Design review of the part built by this model. Coordinates are the model's own, in mm. Face numbers are marked on the shaded views. A direction names the side the tool comes from. Give positions to 0.01 mm unless a question says otherwise; leave off trailing zeros. Loops run counter-clockwise (first coordinate to the right, second up) from the corner with the lowest first, then second, coordinate; pieces in that order, holes last. Notation, with made-up numbers: (9.25, -21.5) - (43.25, -21.5) arc R13 ccw to (43.25, -4.5) - close; hole circle Ø11 at (-32.75, -24.75). An arc over 180 degrees is marked (long way). Write each question's results on one line, items separated by ' | '.
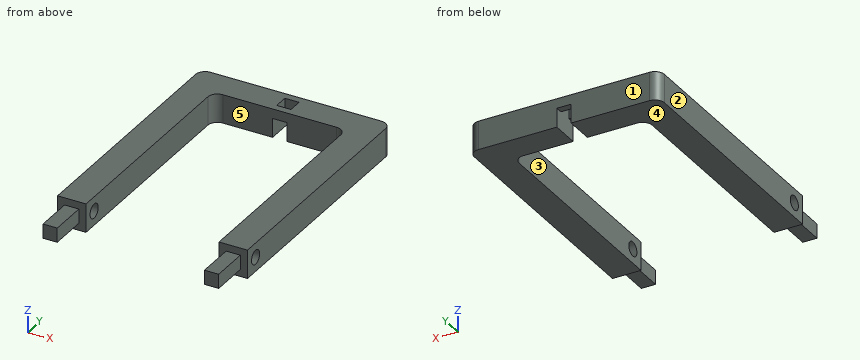
from build123d import *

# Parameters (mm, degrees)
BOSS_EXTRUDE1_DEPTH     = 30
SKETCH2_W               = 15
SKETCH2_H               = 15
BOSS_EXTRUDE2_DEPTH     = 40
FILLET1_R               = 10
FILLET2_R               = 10
SKETCH3_R               = 7.5
CUT_EXTRUDE1_DEPTH      = 171
CUT_EXTRUDE1_DEPTH_BACK = 31
SKETCH4_W               = 15
SKETCH4_H               = 30
CUT_EXTRUDE2_DEPTH      = 20
SKETCH5_W               = 15
SKETCH5_H               = 15
CUT_EXTRUDE3_DEPTH      = 10


with BuildPart() as part:
    # Sketch1 → Boss-Extrude1 (new body)
    with BuildSketch(Plane.XY):
        Polygon((-77.931034483, -87.881800857), (-107.931034483, -87.881800857), (-107.931034483, 177.118199143), (92.068965517, 177.118199143), (92.068965517, -87.881800857), (62.068965517, -87.881800857), (62.068965517, 147.118199143), (-77.931034483, 147.118199143), align=None)
    extrude(amount=BOSS_EXTRUDE1_DEPTH)

    # Sketch2 → Boss-Extrude2 (add)
    with BuildSketch(Plane.XZ.offset(87.881800857)):
        with Locations((77.068965517, 15)):
            Rectangle(SKETCH2_W, SKETCH2_H)
        with Locations((-92.931034483, 15)):
            Rectangle(SKETCH2_W, SKETCH2_H)
    extrude(amount=BOSS_EXTRUDE2_DEPTH)

    # Fillet1
    fillet1_edges = [part.edges().sort_by_distance(p)[0] for p in [
        (62.068965517, 147.118199143, 15),
        (-77.931034483, 147.118199143, 15),
    ]]
    fillet(fillet1_edges, radius=FILLET1_R)

    # Fillet2
    fillet2_edges = [part.edges().sort_by_distance(p)[0] for p in [
        (-107.931034483, 177.118199143, 15),
        (92.068965517, 177.118199143, 15),
    ]]
    fillet(fillet2_edges, radius=FILLET2_R)

    # Sketch3 → Cut-Extrude1 (cut, two sides)
    with BuildSketch(Plane(origin=(-77.931034483, 0, 0), x_dir=(0, 0, -1), z_dir=(1, 0, 0))) as cut_extrude1_sk:
        with Locations((-15, -72.881800857)):
            Circle(SKETCH3_R)
    extrude(amount=CUT_EXTRUDE1_DEPTH, mode=Mode.SUBTRACT)
    extrude(cut_extrude1_sk.sketch, amount=-CUT_EXTRUDE1_DEPTH_BACK, mode=Mode.SUBTRACT)

    # Sketch4 → Cut-Extrude2 (cut)
    with BuildSketch(Plane(origin=(0, 0, 0), x_dir=(-1, 0, 0), z_dir=(0, 0, -1))):
        with Locations((7.930867489, 162.118199143)):
            Rectangle(SKETCH4_W, SKETCH4_H)
    extrude(amount=-CUT_EXTRUDE2_DEPTH, mode=Mode.SUBTRACT)

    # Sketch5 → Cut-Extrude3 (cut)
    with BuildSketch(Plane.XY.offset(30)):
        with Locations((-7.930867489, 162.118199143)):
            Rectangle(SKETCH5_W, SKETCH5_H)
    extrude(amount=-CUT_EXTRUDE3_DEPTH, mode=Mode.SUBTRACT)


solid = part.part
(1) Take a section at A-A on y = -15.5. Give the boundary of the cut face in (x, z).
Answers below:
outline: (-107.93, 0) - (-77.93, 0) - (-77.93, 30) - (-107.93, 30) - close; (62.07, 0) - (92.07, 0) - (92.07, 30) - (62.07, 30) - close
(2) Take a section at C-C on x = -27. Give the boundary of the cut face in (y, z), plus the area to 3 significant figures.
Answers below:
outline: (147.12, 0) - (177.12, 0) - (177.12, 30) - (147.12, 30) - close | area: 900 mm2
(3) Take a section at B-B on z = 15. Count the separate pieces of the cut face and the enclosed holes in it, plus the area to 4 significant figures.
Answers below:
separate pieces: 4 | enclosed holes: 0 | area: 19,950 mm2
(4) Tool access review of the marked faces 4 and 5: name each direction out of +Z, -Z, +X, -X, +Y, -Y from which nothing blocks a thin tool from reaching the whole face with its end or side.
Answers below:
face 4: -Z, +X, -X, +Y, -Y | face 5: +Z, -Z, -Y
(5) Wall thickness on line 1 along Y through (x, z) = (83.25, 15); line 2 along X through (y, z) = (-30, 25.5); line 3 along Y through (x, z) = (-86.5, 15): over which ranges is each line inside the solid? List them lowest first. Write a range as from..to.
Answers below:
line 1: -127.88..-80.38, -65.38..177.05 | line 2: -107.93..-77.93, 62.07..92.07 | line 3: -127.88..-80.38, -65.38..177.12
(6) Draft analysis for pull direction X (two halves, no side actions). For the marked faces 1, 2 and 3, state which applies: pulls with the +X half, pulls with the -X half, needs draft (parallel to the pull), parting line crosses it, or undercut.
Answers below:
face 1: needs draft | face 2: pulls with the -X half | face 3: undercut
(7) Insertion check: P1, Ø16.5, axis at x = 78.5, y = -111, coming from the -Z side; P2, Ø2, axis at x = -7, y = 150, coming from the -Z side; P3, Ø7.5, axis at x = -94.5, y = -107.5, coming from the +Z side; P4, Ø12, axis at y = -72.88, z = 15, coming from the +X side. Each pin has a flat end and moves straight along its axis. Give the tip position at first contact, or say it passes through.
Answers below:
P1: z = 7.5 | P2: z = 20 | P3: z = 22.5 | P4: through
